Autodesk Inventor part; units mm, degrees
ref_plane "YZ Plane" through (0, 0, 0) normal (1, 0, 0) x (0, 1, 0)
ref_plane "XZ Plane" through (0, 0, 0) normal (0, 1, 0) x (-1, 0, 0)
ref_plane "XY Plane" through (0, 0, 0) normal (0, 0, 1) x (1, 0, 0)
sketch "Sketch1" plane through (0, 0, 0) normal (0, 1, 0) x (-1, 0, 0)
  line L0 (21.9604, 29.5602) -> (-24.0396, 29.5602)
  line L1 (-24.0396, 29.5602) -> (-24.0396, -29.4398)
  line L2 (-24.0396, -29.4398) -> (21.9604, -29.4398)
  line L3 (21.9604, -29.4398) -> (21.9604, 29.5602)
  dimension "d0" = 46
  dimension "d1" = 59
extrude "Extrusion1" add sketch "Sketch1" along normal blind 11
sketch "Sketch2" plane through (0, 11, 0) normal (0, 1, 0) x (1, 0, 0)
  line L0 (-18.9604, -32.4344) -> (-8.9604, -32.4344)
  line L1 (-8.9604, -32.4344) -> (-8.9604, 37.5656)
  line L2 (-8.9604, 37.5656) -> (-18.9604, 37.5656)
  line L3 (-18.9604, 37.5656) -> (-18.9604, -32.4344)
  line L4 (-21.9604, 29.4398) -> (-21.9604, -29.5602)
  point P0 (0, 0)
  dimension "d4" = 10
  dimension "d5" = 70
  dimension "d6" = 3
extrude "Extrusion2" cut sketch "Sketch2" against normal blind 8
sketch "Sketch3" plane through (0, 11, 0) normal (0, 1, 0) x (1, 0, 0)
  line L0 (17.0396, -31.142) -> (21.0396, -31.142)
  line L1 (21.0396, -31.142) -> (21.0396, 38.858)
  line L2 (21.0396, 38.858) -> (17.0396, 38.858)
  line L3 (17.0396, 38.858) -> (17.0396, -31.142)
  line L4 (24.0396, -29.5602) -> (24.0396, 29.4398)
  point P0 (0, 0)
  dimension "d9" = 4
  dimension "d10" = 70
  dimension "d11" = 3
extrude "Extrusion3" cut sketch "Sketch3" against normal blind 7
sketch "Sketch4" plane through (0, 3, 0) normal (0, 1, 0) x (1, 0, 0)
  line L0 (-15.9604, -24.5602) -> (-15.9604, -9.5602)
  line L1 (-11.9604, -24.5602) -> (-11.9604, -9.5602)
  arc A0 (-11.9604, -9.5602) -> (-15.9604, -9.5602) centre (-13.9604, -9.5602) ccw
  arc A1 (-15.9604, -24.5602) -> (-11.9604, -24.5602) centre (-13.9604, -24.5602) ccw
  line L2 (-18.9604, -29.5602) -> (-18.9604, 29.4398)
  line L3 (-8.9604, 29.4398) -> (-8.9604, -29.5602)
  line L4 (-8.9604, -29.5602) -> (-18.9604, -29.5602)
  line L5 (-15.9604, 9.4398) -> (-15.9604, 24.4398)
  line L6 (-11.9604, 9.4398) -> (-11.9604, 24.4398)
  arc A2 (-11.9604, 24.4398) -> (-15.9604, 24.4398) centre (-13.9604, 24.4398) ccw
  arc A3 (-15.9604, 9.4398) -> (-11.9604, 9.4398) centre (-13.9604, 9.4398) ccw
  line L7 (-18.9604, 29.4398) -> (-8.9604, 29.4398)
  point P0 (0, 0)
  point P1 (-13.9604, 29.4398)
  point P2 (-11.9604, 16.9398)
  point P3 (-15.9604, 16.9398)
  dimension "d14" = 4
  dimension "d21" = 3
  dimension "d22" = 3
  dimension "d31" = 5
  dimension "d32" = 15
  dimension "d43" = 15
  dimension "d44" = 5
  dimension "d45" = 4
  dimension "d46" = 3
  dimension "d47" = 3
extrude "Extrusion4" add sketch "Sketch4" along normal blind 7 contours L0 A0 L1 A1 | L5 A2 L6 A3
sketch "Sketch6" plane through (0, 10, 0) normal (0, 1, 0) x (1, 0, 0)
  line L0 (-19.9604, -23.5602) -> (-7.9604, -23.5602)
  line L1 (-7.9604, -23.5602) -> (-7.9604, -9.5602)
  line L2 (-7.9604, -9.5602) -> (-19.9604, -9.5602)
  line L3 (-19.9604, -9.5602) -> (-19.9604, -23.5602)
  arc A0 (-11.9604, -9.5602) -> (-15.9604, -9.5602) centre (-13.9604, -9.5602) ccw
  line L4 (-15.9604, -9.5602) -> (-15.9604, -24.5602)
  line L5 (-18.9604, -29.5602) -> (-18.9604, 29.4398)
  line L6 (-8.9604, 29.4398) -> (-8.9604, -29.5602)
  line L7 (-19.9604, 9.4398) -> (-19.9604, 23.4398)
  line L8 (-19.9604, 23.4398) -> (-7.9604, 23.4398)
  line L9 (-7.9604, 23.4398) -> (-7.9604, 9.4398)
  line L10 (-7.9604, 9.4398) -> (-19.9604, 9.4398)
  point P0 (0, 0)
  point P1 (-13.9604, -7.5602)
  point P2 (-19.9604, -16.5602)
  point P3 (-7.9604, 16.4398)
  point P4 (-19.9604, 16.4398)
  point P5 (-18.9604, 9.4398)
  point P6 (-8.9604, 9.4398)
  point P7 (-8.9604, 23.4398)
  point P8 (-18.9604, 23.4398)
  dimension "d33" = 14
  dimension "d35" = 0
  dimension "d37" = 1
  dimension "d41" = 12
  dimension "d48" = 14
  dimension "d49" = 12
  dimension "d62" = 19
extrude "Extrusion6" add sketch "Sketch6" along normal blind 1 contours L3 L2 L5 L0 | L5 L2 L4 L0 | L4 L2 L6 L0 | L6 L2 L1 L0 | L5 L8 L6 L10
sketch "Sketch8" plane through (0, 0, 0) normal (0, -1, 0) x (1, 0, 0)
  line L0 (5.7896, 31.0602) -> (-3.7104, 31.0602)
  line L1 (-3.7104, 31.0602) -> (-3.7104, -30.9398)
  line L2 (-3.7104, -30.9398) -> (5.7896, -30.9398)
  line L3 (5.7896, -30.9398) -> (5.7896, 31.0602)
  line L4 (-21.9604, 29.5602) -> (24.0396, 29.5602)
  line L5 (24.0396, -29.4398) -> (-21.9604, -29.4398)
  line L6 (24.0396, 29.5602) -> (24.0396, -29.4398)
  line L7 (-21.9604, -29.4398) -> (-21.9604, 29.5602)
  point P0 (0, 0)
  point P1 (-3.7104, -29.4398)
  point P2 (5.7896, -29.4398)
  point P3 (5.7896, 29.5602)
  point P4 (-3.7104, 29.5602)
  dimension "d50" = 9.5
  dimension "d51" = 62
  dimension "d52" = 1.5
  dimension "d53" = 1.5
  dimension "d54" = 18.25
  dimension "d55" = 18.25
extrude "Extrusion7" add sketch "Sketch8" along normal blind 6 contours L3 L5 L1 L4
sketch "Sketch9" plane through (24.0396, 0, -29.4398) normal (0, 0, -1) x (-1, 0, 0)
  point P0 (24.0396, 0)
sketch "Sketch10" plane through (24.0396, 0, -29.4398) normal (0, 0, -1) x (-1, 0, 0)
  line L0 (0, 0) -> (18.25, 0)
  line L1 (27.75, 0) -> (27.75, -6)
  line L2 (18.25, 0) -> (27.75, 0)
  line L3 (27.75, 0) -> (27.75, -6)
  line L4 (27.75, -6) -> (18.25, -6)
  line L5 (18.25, -6) -> (18.25, 0)
  point P0 (24.0396, 0)
extrude "Extrusion8" add sketch "Sketch10" along normal blind 10
sketch "Sketch11" plane through (-21.9604, 0, 29.5602) normal (0, 0, 1) x (1, 0, 0)
  line L0 (0, 0) -> (18.25, 0)
  line L1 (18.25, 0) -> (27.75, 0)
  line L2 (27.75, 0) -> (27.75, -6)
  line L3 (27.75, -6) -> (18.25, -6)
  line L4 (18.25, -6) -> (18.25, 0)
  point P0 (21.9604, 0)
extrude "Extrusion9" add sketch "Sketch11" along normal blind 10
sketch "Sketch12" plane through (0, 11, 0) normal (0, 1, 0) x (1, 0, 0)
  line L0 (24.0396, -29.5602) -> (24.0396, 29.4398)
  line L1 (-21.9604, 29.4398) -> (-21.9604, -29.5602)
  line L2 (24.0396, -29.5602) -> (-21.9604, -29.5602)
  line L3 (-21.9604, -29.5602) -> (-21.9604, -23.5602)
  line L4 (24.0396, -23.5602) -> (24.0396, -29.5602)
  line L5 (-21.9604, 29.4398) -> (24.0396, 29.4398)
  line L6 (24.0396, 29.4398) -> (24.0396, 23.4398)
  line L7 (-21.9604, 23.4398) -> (-21.9604, 29.4398)
  line L8 (-21.9604, -23.5602) -> (-3.6341, -23.5602)
  line L9 (5.8705, -23.5602) -> (24.0396, -23.5602)
  line L10 (24.0396, 23.4398) -> (5.8705, 23.4398)
  line L11 (-3.6341, 23.4398) -> (-21.9604, 23.4398)
  line L12 (-3.6341, 29.4398) -> (-3.6341, 23.4398)
  line L13 (-3.6341, -23.5602) -> (-3.6341, -29.5602)
  line L14 (5.8705, -29.5602) -> (5.8705, -23.5602)
  line L15 (5.8705, 23.4398) -> (5.8705, 29.4398)
  point P0 (0, 0)
  point P1 (-21.9604, -29.5602)
  dimension "d63" = 6
  dimension "d64" = 6
extrude "Extrusion10" cut sketch "Sketch12" against normal blind 100 contours L2 L14 L9 L0 | L10 L15 L5 L0 | L2 L1 L8 L13 | L12 L11 L1 L5
properties part number "table_bridge"
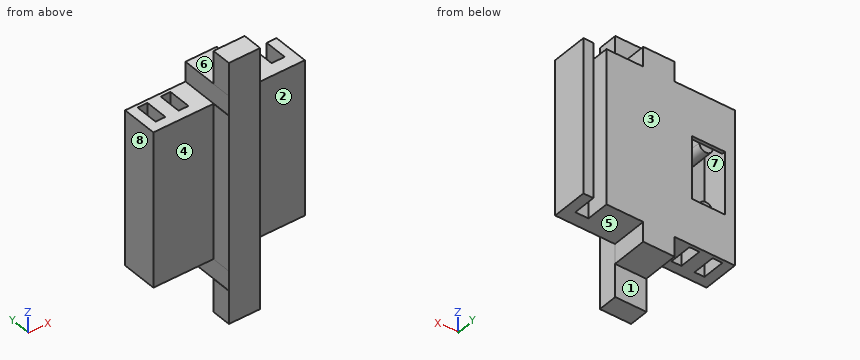
Can you work these out from the model? Positions are in its coordinate system, mm. Face numbers are marked on the shaded views. A direction names the side the tool comes from. Round coordinates to 2 decimals unless told otherwise and drop trailing zeros. Order: outer loops, then holes, each group sorted by start corner. A loop starts at its lowest first (then second) coordinate and runs counter-clockwise, first axis right, second up. Notation, with made-up numbers: (-2, 56) -> (33, 56) arc R27 ccw to (33, 90) -> close; hole circle Ø6 at (63.25, 62). An arc over 180 degrees is marked (long way). Return JSON: item names as keys, results as strings. Group by question number.
1. If we section it at B-B, the plane z = 21.5: Write out the boundary of the cut face in (x, y), then the cut area to 3 significant figures.
2. We'd pull the mould along X, two halves only. Please class the marked faces 6, 7 and 8: released by +X, released by -X, zero draft, split by the parting line, or undercut.
3. If we section it at A-A, the plane y = 4.75: Write out the boundary of the cut face in (x, z).
4. If we section it at D-D, the plane x = 13: Write out the boundary of the cut face in (y, z), then the cut area to 3 significant figures.
5. If we section it at C-C, the plane z = -5.5: Write out the boundary of the cut face in (x, y), then the cut area to 3 significant figures.
6. Will these pins go through, and if not, where does the flat tip stop? pin 1 (1.8 mm diameter, centred on y = -1.5, z = -32, fed in from -X); pin 2 (20 mm diameter, centred on x = 18.5, z = -9, fed in from -Y); pin 3 (1.5 mm diameter, centred on x = -6.5, y = 4, fed in from +Z).
7. I need wall thicknesses on line 1 (X direction, y = 8.5, z = -18.5); line 2 (Z direction, x = 14, y = 7.25); line 3 (X direction, y = 9, z = 28). Which ranges of each line are inside material? Lowest first, please. Write a range as [from, to].
8. Which directions (+Z, -Z, +X, -X, +Y, -Y) give clear straight access to the entire face, cutting with the end or side of a thin tool? Please do the marked faces 1, 2, 3, 4 and 5.
Output values:
{
 "1": {"outline": "(-21.96, 0) -> (-3.71, 0) -> (-3.71, -6) -> (5.79, -6) -> (5.79, 0) -> (24.04, 0) -> (24.04, 11) -> (21.04, 11) -> (21.04, 4) -> (17.04, 4) -> (17.04, 11) -> (-21.96, 11) -> close; hole (-18.96, 3) -> (-15.96, 3) -> (-15.96, 10) -> (-18.96, 10) -> close; hole (-11.96, 3) -> (-8.96, 3) -> (-8.96, 10) -> (-11.96, 10) -> close", "area": "493 mm²"},
 "2": {"face 6": "zero draft", "face 7": "undercut", "face 8": "released by -X"},
 "3": {"outline": "(-21.96, -23.44) -> (-18.96, -23.44) -> (-18.96, 23.56) -> (-21.96, 23.56) -> close; (-15.96, -23.44) -> (-11.96, -23.44) -> (-11.96, -9.44) arc R2 ccw to (-15.96, -9.44) -> close; (-15.96, 9.56) arc R2 ccw to (-11.96, 9.56) -> (-11.96, 23.56) -> (-15.96, 23.56) -> close; (-8.96, -23.44) -> (-3.63, -23.44) -> (-3.63, -29.44) -> (5.87, -29.44) -> (5.87, -23.44) -> (17.04, -23.44) -> (17.04, 23.56) -> (5.87, 23.56) -> (5.87, 29.56) -> (-3.63, 29.56) -> (-3.63, 23.56) -> (-8.96, 23.56) -> close; (21.04, -23.44) -> (24.04, -23.44) -> (24.04, 23.56) -> (21.04, 23.56) -> close"},
 "4": {"outline": "(0, -23.44) -> (11, -23.44) -> (11, 23.56) -> (0, 23.56) -> close", "area": "517 mm²"},
 "5": {"outline": "(-21.96, 0) -> (-3.71, 0) -> (-3.71, -6) -> (5.79, -6) -> (5.79, 0) -> (24.04, 0) -> (24.04, 11) -> (21.04, 11) -> (21.04, 4) -> (17.04, 4) -> (17.04, 11) -> (-8.96, 11) -> (-8.96, 3) -> (-18.96, 3) -> (-18.96, 11) -> (-21.96, 11) -> close", "area": "455 mm²"},
 "6": {"pin 1": "x = -3.71", "pin 2": "y = 0", "pin 3": "z = 23.56"},
 "7": {"line 1": "[-21.96, -18.96], [-15.96, -11.96], [-8.96, 17.04], [21.04, 24.04]", "line 2": "[-23.44, 23.56]", "line 3": "[-3.63, 5.87]"},
 "8": {"face 1": "-Z, +X, -X, +Y", "face 2": "+Z, -Z, +X, -Y", "face 3": "+Z, -Z, +X, -X, +Y", "face 4": "+Z, -Z, -X, -Y", "face 5": "-Z, +X, +Y, -Y"}
}
